from build123d import *

# Parameters (mm, degrees)
EXTRUDE_1_DEPTH = 1


with BuildPart() as part:
    # 草图1 → 凸台-拉伸1 (new body)
    with BuildSketch(Plane.XY):
        with BuildLine():
            Line((15.51403903, -5.321145834), (1.163677412, 16.35988554))
            ThreePointArc((1.163677412, 16.35988554), (-0.105358364, 17.215860979), (-1.607968203, 16.923783214))
            Line((-1.607968203, 16.923783214), (-14.950141356, 8.092791449))
            ThreePointArc((-14.950141356, 8.092791449), (-15.806116795, 6.823755673), (-15.51403903, 5.321145834))
            Line((-15.51403903, 5.321145834), (-1.163677412, -16.35988554))
            ThreePointArc((-1.163677412, -16.35988554), (0.105358364, -17.215860979), (1.607968203, -16.923783214))
            Line((1.607968203, -16.923783214), (14.950141356, -8.092791449))
            ThreePointArc((14.950141356, -8.092791449), (15.806116795, -6.823755673), (15.51403903, -5.321145834))
        make_face()
        with BuildLine():
            ThreePointArc((11.356570608, -4.475299323), (9.277836397, -4.052376068), (8.854913141, -6.131110279))
            ThreePointArc((8.854913141, -6.131110279), (10.933647352, -6.554033535), (11.356570608, -4.475299323))
        make_face(mode=Mode.SUBTRACT)
        with BuildLine():
            ThreePointArc((2.183826565, -10.546606162), (0.105092354, -10.123682907), (-0.317830901, -12.202417118))
            ThreePointArc((-0.317830901, -12.202417118), (1.76090331, -12.625340373), (2.183826565, -10.546606162))
        make_face(mode=Mode.SUBTRACT)
        with BuildLine():
            ThreePointArc((-8.854913141, 6.131110279), (-10.933647352, 6.554033535), (-11.356570608, 4.475299323))
            ThreePointArc((-11.356570608, 4.475299323), (-9.277836397, 4.052376068), (-8.854913141, 6.131110279))
        make_face(mode=Mode.SUBTRACT)
        with BuildLine():
            ThreePointArc((0.317830901, 12.202417118), (-1.76090331, 12.625340373), (-2.183826565, 10.546606162))
            ThreePointArc((-2.183826565, 10.546606162), (-0.105092354, 10.123682907), (0.317830901, 12.202417118))
        make_face(mode=Mode.SUBTRACT)
    extrude(amount=EXTRUDE_1_DEPTH)


solid = part.part
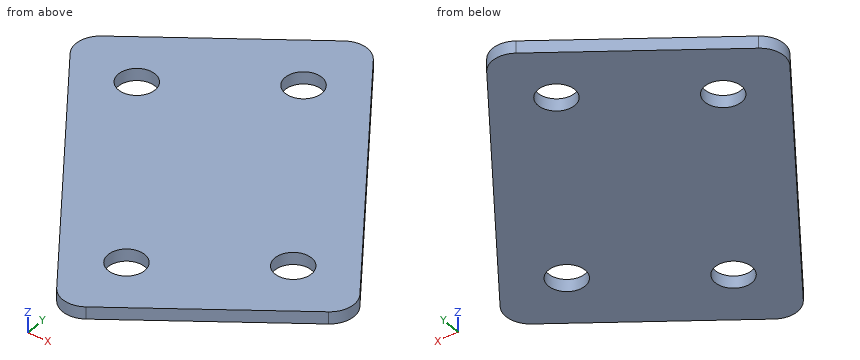
Work out the finished part from the listing and answer in its coordinate system (mm). Coordinates: 2 decimals unless noted, no trailing zeros. Write each loop counter-clockwise with the first axis right and the second up, starting at its lowest first coordinate (ties: lowest second). Pieces come first, ordered by that corner, then holes. Notation, with made-up numbers: M -40,24 L -30,24 A22 ccw -30,43 Z; hole C 55,-34.5 d4. An arc over 180 degrees is marked long. Write item = value, one per line.
1. The part is cut by section A-A (x = -9.5). Determine the outline of the cut face in (y, z), then the cut area to 3 significant figures.
Solution:
outline = M -3.77,0 L 3.93,0 L 3.93,1 L -3.77,1 Z; M 6.68,0 L 11.7,0 L 11.7,1 L 6.68,1 Z
area = 12.7 mm2
2. The part is cut by section B-B (z = 0.3). Determine the outline of the cut face in (x, y).
Solution:
outline = M -15.51,5.32 L -1.16,-16.36 A2 ccw 1.61,-16.92 L 14.95,-8.09 A2 ccw 15.51,-5.32 L 1.16,16.36 A2 ccw -1.61,16.92 L -14.95,8.09 A2 ccw Z; hole C -10.11,5.3 d3; hole C -0.93,11.37 d3; hole C 0.93,-11.37 d3; hole C 10.11,-5.3 d3
3. Straight lines are drawn through the part: line 1 (Y direction, x = 0, z = 0.7); line 2 (X direction, y = 6, z = 0.2); line 3 (Y direction, x = 2.5, z = 0.6). For each, find the intervals that lie inside material, in ascending order. Write a range as from..to.
Solution:
line_1 = -17.19..-12.55, -10.2..10.2, 12.55..17.19
line_2 = -15.8..-11.43, -8.78..8.02
line_3 = -16.33..14.34
4. The part is cut by section D-D (x = -5). Determine the outline of the cut face in (y, z), then the cut area to 3 significant figures.
Solution:
outline = M -10.56,0 L 14.68,0 L 14.68,1 L -10.56,1 Z
area = 25.2 mm2
5. The part is cut by section C-C (y = -1). Determine the outline of the cut face in (x, z).
Solution:
outline = M -11.33,0 L 12.65,0 L 12.65,1 L -11.33,1 Z
